from build123d import *

# Parameters (mm, degrees)
SKETCH1_W           = 35
SKETCH1_H           = 65
BOSS_EXTRUDE1_DEPTH = 2.5
SKETCH2_W           = 4
SKETCH2_H           = 65
BOSS_EXTRUDE2_DEPTH = 38.5
SKETCH3_W           = 31
SKETCH3_H           = 2.5
BOSS_EXTRUDE4_DEPTH = 38.5
BOSS_EXTRUDE6_DEPTH = 11.15
SKETCH15_R          = 2
CUT_EXTRUDE3_DEPTH  = 5
CUT_EXTRUDE6_DEPTH  = 7
BOSS_EXTRUDE7_DEPTH = 6.44


with BuildPart() as part:
    # Sketch1 → Boss-Extrude1 (new body)
    with BuildSketch(Plane(origin=(0, 0, 0), x_dir=(1, 0, 0), z_dir=(0, 1, 0))):
        Rectangle(SKETCH1_W, SKETCH1_H)
    extrude(amount=BOSS_EXTRUDE1_DEPTH)

    # Sketch2 → Boss-Extrude2 (add)
    with BuildSketch(Plane(origin=(0, 2.5, 0), x_dir=(1, 0, 0), z_dir=(0, 1, 0))):
        with Locations((-15.5, 0)):
            Rectangle(SKETCH2_W, SKETCH2_H)
    extrude(amount=BOSS_EXTRUDE2_DEPTH)

    # Sketch3 → Boss-Extrude4 (add)
    with BuildSketch(Plane(origin=(0, 2.5, 0), x_dir=(1, 0, 0), z_dir=(0, 1, 0))):
        with Locations((2, 31.25)):
            Rectangle(SKETCH3_W, SKETCH3_H)
        with Locations((2, -31.25)):
            Rectangle(SKETCH3_W, SKETCH3_H)
    extrude(amount=BOSS_EXTRUDE4_DEPTH)

    # Sketch12 → Boss-Extrude6 (add)
    with BuildSketch(Plane(origin=(0, 41, 0), x_dir=(1, 0, 0), z_dir=(0, 1, 0))):
        Polygon((-8.203844825, -13.796665784), (-9.645047449, -15.79282096), (-10.2, -15.79282096), (-13.5, -15.740186096), (-13.5, -13.717271913), (-10.2, -13.717271913), (-10.2, -10.374022399), (-8.203844825, -10.374022399), align=None)
        Polygon((-13.5, 13.717271913), (-10.2, 13.717271913), (-10.2, 8.874022399), (-8.203844825, 8.874022399), (-8.203844825, 13.796665784), (-9.645047449, 15.721544213), (-13.5, 15.721544213), align=None)
    extrude(amount=-BOSS_EXTRUDE6_DEPTH)

    # Sketch15 → Cut-Extrude3 (cut)
    with BuildSketch(Plane(origin=(0, 2.5, 0), x_dir=(1, 0, 0), z_dir=(0, 1, 0))):
        with Locations(Location((8.550066744, 0, 0), (0, 0, 270))):
            Circle(SKETCH15_R)
    extrude(amount=-CUT_EXTRUDE3_DEPTH, mode=Mode.SUBTRACT)

    # Sketch13 → Cut-Extrude6 (cut)
    with BuildSketch(Plane(origin=(-13.5, 0, 0), x_dir=(0, 0, -1), z_dir=(1, 0, 0))):
        Polygon((-15.719309169, 34.85), (-19.050762409, 34.85), (-19.050762409, 41), (-15.740186096, 41), (21.565915306, 41), (24.332393972, 41), (24.332393972, 34.85), (21.565915306, 34.85), align=None)
    extrude(amount=CUT_EXTRUDE6_DEPTH, mode=Mode.SUBTRACT)

    # Sketch7 → Boss-Extrude7 (add)
    with BuildSketch(Plane(origin=(0, 2.5, 0), x_dir=(1, 0, 0), z_dir=(0, 1, 0))):
        Polygon((-13.5, 13.717271913), (-13.5, 15.696799482), (-9.20372121, 15.696799482), (-8.173305913, 13.796665784), (-8.173305913, 11.874022399), (-8.173305913, 10.367152571), (-10.2, 10.367152571), (-10.2, 13.717271913), align=None)
        Polygon((-13.5, -13.717271913), (-13.5, -15.696799482), (-9.20372121, -15.696799482), (-8.203759602, -13.717271913), (-8.203759602, -10.374022403), (-10.2, -10.374022403), (-10.2, -13.717271913), align=None)
    extrude(amount=BOSS_EXTRUDE7_DEPTH)


solid = part.part
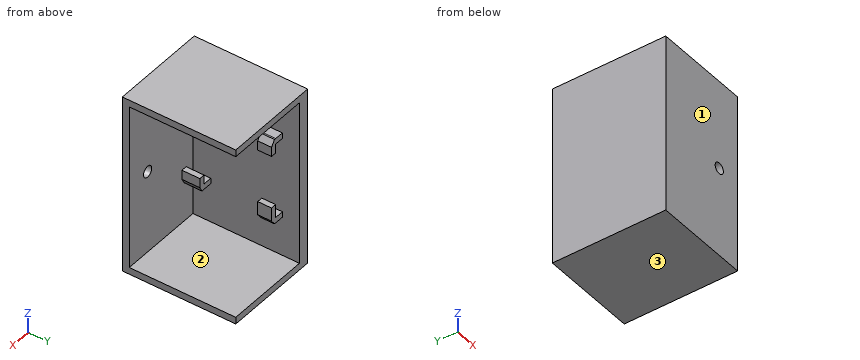
Part model, mm, in its own coordinate system. Face numbers are marked on the shaded views. Coordinates: 2 decimals unless noted, no trailing zeros. Order: outer loops, then holes, each group sorted by start corner. A loop starts at its lowest first (then second) coordinate and runs counter-clockwise, first axis right, second up.
(1) Pin check, flat tips, straight feed: pin 1 Ø2.5 at (y, z) = (31.5, -11.5) entering from +X; pin 2 Ø9.5 at (x, z) = (7, 4.5) entering from +Y; pin 3 Ø2.5 at (x, z) = (-11, 13) entering from +Y. Stop position of each tip, or through.
Check sheet entries:
pin 1: stops at x = -8.2
pin 2: stops at y = 2.5
pin 3: stops at y = 34.85
(2) Slice it at B-B, the plane y = 11.5. Write the cut outline in (x, z), and give its area (3 significant figures).
Check sheet entries:
outline: (-17.5, -32.5) - (17.5, -32.5) - (17.5, -30) - (-13.5, -30) - (-13.5, 30) - (17.5, 30) - (17.5, 32.5) - (-17.5, 32.5) - close
area: 415 mm2
(3) Slice it at A-A, the plane z = 0. Write the cut outline in (x, y), and give its area (4 significant figures).
Check sheet entries:
outline: (-17.5, 0) - (6.55, 0) - (6.55, 2.5) - (-13.5, 2.5) - (-13.5, 41) - (-17.5, 41) - close; (10.55, 0) - (17.5, 0) - (17.5, 2.5) - (10.55, 2.5) - close
area: 231.5 mm2
(4) Slice it at C-C, the plane x = 0.5. Write the cut outline in (y, z), and give its area (3 significant figures).
Check sheet entries:
outline: (0, -32.5) - (41, -32.5) - (41, -30) - (2.5, -30) - (2.5, 30) - (41, 30) - (41, 32.5) - (0, 32.5) - close
area: 355 mm2
(5) Probe L1, parallel to Z at x = -1, y = 31; L2, parallel to Y at x = 1, z = 2.5; L3, parallel to X at y = 1.75, z = 0. List the from-to ranges inside material, lowest first.
Check sheet entries:
L1: z = -32.5 to -30, 30 to 32.5
L2: y = 0 to 2.5
L3: x = -17.5 to 6.55, 10.55 to 17.5
(6) Pull direction Z, two halves, no side cores. Call the marked faces 1, 2 and 3: pulls with the +Z half, pulls with the -Z half, needs draft (parallel to the pull), parting line crosses it, or undercut.
Check sheet entries:
face 1: needs draft
face 2: undercut
face 3: pulls with the -Z half
(7) Slice it at D-D, the plane z = -22.5. Write the cut outline in (x, y).
Check sheet entries:
outline: (-17.5, 0) - (17.5, 0) - (17.5, 2.5) - (-13.5, 2.5) - (-13.5, 41) - (-17.5, 41) - close
